Source: CAD feature listing. Evaluate the final solid. Frame: model axes, mm. Give positions to 0.01 mm unless a question says otherwise; leave off trailing zeros. Write each loop counter-clockwise with the first axis right and the second up, starting at its lowest first coordinate (ties: lowest second). Pieces come first, ordered by that corner, then holes.
Autodesk Inventor part; units mm, degrees
ref_plane "Plan médian largeur" through (-65.6569, 0, -27.413) normal (0, 0, 1) x (1, 0, 0)
ref_plane "YZ Plane" through (0, 0, 0) normal (1, 0, 0) x (0, 1, 0)
ref_plane "XZ Plane" through (0, 0, 0) normal (0, 1, 0) x (-1, 0, 0)
sketch "Esquisse1" plane through (0, 0, 0) normal (0, 1, 0) x (-1, 0, 0)
  line L0 (65.6569, 117.587) -> (-26.3431, 117.587)
  line L1 (-26.3431, 117.587) -> (-26.3431, -172.413)
  line L2 (-26.3431, -172.413) -> (65.6569, -172.413)
  line L3 (65.6569, -172.413) -> (65.6569, 117.587)
  line L4 (55.6569, 69.587) -> (-16.3431, 69.587)
  line L5 (-18.3431, 67.587) -> (-18.3431, 41.587)
  line L6 (-16.3431, 39.587) -> (55.6569, 39.587)
  line L7 (57.6569, 41.587) -> (57.6569, 67.587)
  arc A0 (-18.3431, 41.587) -> (-16.3431, 39.587) centre (-16.3431, 41.587) ccw
  arc A1 (55.6569, 39.587) -> (57.6569, 41.587) centre (55.6569, 41.587) ccw
  arc A2 (57.6569, 67.587) -> (55.6569, 69.587) centre (55.6569, 67.587) ccw
  arc A3 (-16.3431, 69.587) -> (-18.3431, 67.587) centre (-16.3431, 67.587) ccw
  line L8 (65.6569, -27.413) -> (-26.3431, -27.413) construction
  line L9 (55.6569, -124.413) -> (-16.3431, -124.413)
  line L10 (-18.3431, -122.413) -> (-18.3431, -96.413)
  line L11 (-16.3431, -94.413) -> (55.6569, -94.413)
  line L12 (57.6569, -96.413) -> (57.6569, -122.413)
  arc A4 (-16.3431, -94.413) -> (-18.3431, -96.413) centre (-16.3431, -96.413) ccw
  arc A5 (57.6569, -96.413) -> (55.6569, -94.413) centre (55.6569, -96.413) ccw
  arc A6 (55.6569, -124.413) -> (57.6569, -122.413) centre (55.6569, -122.413) ccw
  arc A7 (-18.3431, -122.413) -> (-16.3431, -124.413) centre (-16.3431, -122.413) ccw
  point P0 (0, 0)
  dimension "d0" = 290
  dimension "d1" = 92
  dimension "d7" = 30
  dimension "d8" = 8
  dimension "d9" = 8
  dimension "d10" = 2
  dimension "d15" = 48
  dimension "d23" = 145
extrude "Extrusion1" add sketch "Esquisse1" along normal blind 4
sketch "Esquisse3" plane through (0, 4, 0) normal (0, 1, 0) x (1, 0, 0)
  circle A0 centre (-35.2599, -31.2495) radius 1.5875
  circle A1 centre (-35.2599, -18.5495) radius 1.5875
  circle A2 centre (-35.2599, -5.8495) radius 1.5875
  arc A3 (-57.6569, 96.413) -> (-55.6569, 94.413) centre (-55.6569, 96.413) ccw
  line L0 (-57.6569, 96.413) -> (-57.6569, 122.413)
  arc A4 (-55.6569, 124.413) -> (-57.6569, 122.413) centre (-55.6569, 122.413) ccw
  line L1 (-55.6569, 124.413) -> (16.3431, 124.413)
  arc A5 (18.3431, 122.413) -> (16.3431, 124.413) centre (16.3431, 122.413) ccw
  line L2 (18.3431, 122.413) -> (18.3431, 96.413)
  arc A6 (16.3431, 94.413) -> (18.3431, 96.413) centre (16.3431, 96.413) ccw
  line L3 (16.3431, 94.413) -> (-55.6569, 94.413)
  arc A7 (16.3431, -69.587) -> (18.3431, -67.587) centre (16.3431, -67.587) ccw
  line L4 (16.3431, -69.587) -> (-55.6569, -69.587)
  arc A8 (-57.6569, -67.587) -> (-55.6569, -69.587) centre (-55.6569, -67.587) ccw
  line L5 (-57.6569, -67.587) -> (-57.6569, -41.587)
  arc A9 (-55.6569, -39.587) -> (-57.6569, -41.587) centre (-55.6569, -41.587) ccw
  line L6 (-55.6569, -39.587) -> (16.3431, -39.587)
  arc A10 (18.3431, -41.587) -> (16.3431, -39.587) centre (16.3431, -41.587) ccw
  line L7 (18.3431, -41.587) -> (18.3431, -67.587)
  line L8 (-65.6569, -117.587) -> (26.3431, -117.587)
  line L9 (26.3431, -117.587) -> (26.3431, 172.413)
  line L10 (26.3431, 172.413) -> (-65.6569, 172.413)
  line L11 (-65.6569, 172.413) -> (-65.6569, -117.587)
  circle A11 centre (-35.2599, 6.8505) radius 1.5875
  circle A12 centre (-4.0179, -31.2495) radius 1.5875
  circle A13 centre (-4.0179, -18.5495) radius 1.5875
  circle A14 centre (-4.0179, -5.8495) radius 1.5875
  circle A15 centre (-4.0179, 6.8505) radius 1.5875
extrude "Extrusion3" cut sketch "Esquisse3" against normal through all contours A0 | A1 | A2 | A11 | A12 | A13 | A14 | A15
ref_plane "Plan médian largeur" through (-65.6569, 0, -27.413) normal (0, 0, 1) x (1, 0, 0)
sketch "Esquisse4" plane through (0, 4, 0) normal (0, 1, 0) x (1, 0, 0)
  line L0 (-2.6569, -69.587) -> (-2.6569, -111.587)
  line L1 (16.3431, -69.587) -> (-55.6569, -69.587)
  line L2 (-36.6569, -69.587) -> (-36.6569, -111.587)
  line L3 (-65.6569, 172.413) -> (-65.6569, -117.587)
  line L4 (-34.6569, -113.587) -> (-4.6569, -113.587)
  arc A0 (-36.6569, -111.587) -> (-34.6569, -113.587) centre (-34.6569, -111.587) ccw
  arc A1 (-4.6569, -113.587) -> (-2.6569, -111.587) centre (-4.6569, -111.587) ccw
  point P0 (0, 0)
  point P1 (-36.6569, -113.587)
  dimension "d52" = 2
  dimension "d53" = 29
  dimension "d67" = 34
extrude "Extrusion4" cut sketch "Esquisse4" against normal through all
sketch "Esquisse6" plane through (0, 0, 0) normal (0, -1, 0) x (1, 0, 0)
  circle A0 centre (-61.6569, 113.587) radius 1.5
  circle A1 centre (22.3431, 113.587) radius 1.5
  circle A2 centre (22.3431, 35.587) radius 1.5
  circle A3 centre (-61.6569, 35.587) radius 1.5
  circle A4 centre (-61.6569, -27.413) radius 1.5
  circle A5 centre (22.3431, -27.413) radius 1.5
  line L0 (-65.6569, -172.413) -> (-65.6569, 117.587)
  line L1 (-65.6569, 117.587) -> (26.3431, 117.587)
  line L2 (26.3431, 117.587) -> (26.3431, -172.413)
  line L3 (16.3431, 39.587) -> (-55.6569, 39.587)
  point P0 (0, 0)
  dimension "d32" = 3
  dimension "d33" = 3
  dimension "d34" = 3
  dimension "d35" = 3
  dimension "d36" = 3
  dimension "d37" = 3
  dimension "d38" = 4
  dimension "d39" = 4
  dimension "d40" = 4
  dimension "d41" = 4
  dimension "d42" = 4
  dimension "d43" = 4
  dimension "d44" = 4
  dimension "d45" = 4
  dimension "d46" = 4
  dimension "d47" = 145
  dimension "d48" = 145
  dimension "d49" = 4
extrude "Extrusion5" cut sketch "Esquisse6" against normal through all
sketch "Esquisse7" plane through (0, 4, 0) normal (0, 1, 0) x (1, 0, 0)
  circle A0 centre (11.3431, -95.587) radius 1.9
  circle A1 centre (11.3431, -85.587) radius 1.9
  circle A2 centre (6.3431, -90.587) radius 4.25
  circle A3 centre (-40.6569, -95.587) radius 1.9
  circle A4 centre (1.3431, -95.587) radius 1.9
  circle A5 centre (1.3431, -85.587) radius 1.9
  circle A6 centre (11.3431, -95.587) radius 1.5
  circle A7 centre (1.3431, -95.587) radius 1.5
  circle A8 centre (6.3431, -90.587) radius 2.5
  circle A9 centre (1.3431, -85.587) radius 1.5
  circle A10 centre (11.3431, -85.587) radius 1.5
  circle A11 centre (-50.6569, -95.587) radius 1.5
  circle A12 centre (-50.6569, -85.587) radius 1.5
  circle A13 centre (-40.6569, -85.587) radius 1.5
  circle A14 centre (-45.6569, -90.587) radius 2.75
  circle A15 centre (-40.6569, -95.587) radius 1.5
  circle A16 centre (-50.6569, -95.587) radius 1.5
  circle A17 centre (-50.6569, -85.587) radius 1.5
  circle A18 centre (-40.6569, -85.587) radius 1.5
  circle A19 centre (-45.6569, -90.587) radius 2.5
  line L0 (-2.6569, -69.587) -> (-2.6569, -111.587)
  line L1 (-65.6569, -117.587) -> (26.3431, -117.587)
  line L2 (-36.6569, -111.587) -> (-36.6569, -69.587)
  point P0 (0, 0)
  dimension "d55" = 3
  dimension "d56" = 3
  dimension "d57" = 5
  dimension "d58" = 3
  dimension "d59" = 3
  dimension "d60" = 3
  dimension "d61" = 3
  dimension "d62" = 3
  dimension "d63" = 3
  dimension "d64" = 5
  dimension "d72" = 8.5
  dimension "d73" = 3.8
  dimension "d74" = 3.8
  dimension "d75" = 3.8
  dimension "d76" = 3.8
  dimension "d77" = 10
  dimension "d78" = 10
  dimension "d79" = 10
  dimension "d80" = 10
  dimension "d81" = 5
  dimension "d82" = 5
  dimension "d83" = 9
  dimension "d84" = 27
  dimension "d85" = 5
  dimension "d86" = 5
  dimension "d87" = 3.8
  dimension "d88" = 5.5
  dimension "d89" = 5
  dimension "d90" = 10
  dimension "d91" = 5
  dimension "d92" = 5
  dimension "d93" = 10
  dimension "d94" = 9
  dimension "d95" = 5
  dimension "d96" = 10
  dimension "d97" = 10
  dimension "d98" = 27
extrude "Extrusion6" cut sketch "Esquisse7" against normal through all contours A6 | A7 | A8 | A9 | A10 | A11 | A12 | A13 | A15 | A19
mirror "Symétrie1" about plane through (-65.6569, 0, -27.413) normal (0, 0, 1) of "Extrusion3", "Extrusion4", "Extrusion5", "Extrusion6"
fillet "Congé1" radius 2 1 edges at (-2.6569, 2, 69.587)
fillet "Congé2" radius 2 1 edges at (-36.6569, 2, 69.587)
fillet "Congé3" radius 2 1 edges at (-2.6569, 2, -124.413)
fillet "Congé4" radius 2 1 edges at (-36.6569, 2, -124.413)
equation "\"d23\" = 0.5 * d0"
properties part number "socle_ammovible"
1. Section query A-A (z = 61). Return loops of the section in (x, y).
2. Pull-direction query (Z, two-part tool) for faces 1 (the flat face through (-19, 0, -25)), 2 (the cylindrical face through (-43.27, 2.03, 89.84)); classes: pulls with the +Z half, pulls with the -Z half, needs draft (parallel to the pull), parting line crosses it, or undercut.
3. Line query: probe 1 along Z at (x, y) = (-31, 1.95); probe 2 along Z at (x, y) = (-43, 1.85); probe 3 along X at (y, z) = (0.35, 75.5). Output: solid intervals per line, ascending.
4. Pin query (flat end, axial travel): P1, Ø3.5, axis at x = 22.34, z = -168.41, coming from the +Y side. Return the tip coordinate at first contact, or that it passes through.
5. Section query B-B (x = -13.5). Return loops of the section in (y, z).
6. Section query C-C (z = -129.5). Return loops of the section in (x, y), plus the area to 3 significant figures.
7. Section query D-D (y = 1.95). Give the number of separate pieces and of enclosed holes in the cut face, plus the area to 3 significant figures.
The answers:
1. outline: (-65.66, 0) - (-57.66, 0) - (-57.66, 4) - (-65.66, 4) - close; (18.34, 0) - (26.34, 0) - (26.34, 4) - (18.34, 4) - close
2. face 1: needs draft
2. face 2: undercut
3. probe 1: z = -172.41 to -168.41, -94.41 to 39.59, 113.59 to 117.59
3. probe 2: z = -172.41 to -124.41, -94.41 to 39.59, 69.59 to 117.59
3. probe 3: x = -65.66 to -36.66, -2.66 to 26.34
4. P1: stops at y = 4
5. outline: (0, -172.41) - (4, -172.41) - (4, -168.41) - (0, -168.41) - close; (0, -94.41) - (4, -94.41) - (4, 39.59) - (0, 39.59) - close; (0, 113.59) - (4, 113.59) - (4, 117.59) - (0, 117.59) - close
6. outline: (-65.66, 0) - (-36.66, 0) - (-36.66, 4) - (-65.66, 4) - close; (-2.66, 0) - (26.34, 0) - (26.34, 4) - (-2.66, 4) - close
6. area: 232 mm2
7. separate pieces: 1
7. enclosed holes: 48
7. area: 18,700 mm2
